Verification items for the finished model (mm, model axes). Give positions to 0.01 mm unless a question says otherwise; leave off trailing zeros. Order: outer loops, then holes, each group sorted by start corner. A loop starts at its lowest first (then second) coordinate and runs counter-clockwise, first axis right, second up.
from build123d import *

# Parameters (mm, degrees)
F0_R     = 116
F1_DEPTH = 6
F3_D     = 9.1
F5_D     = 23


with BuildPart() as f1:
    # F0 (on Top) → F1 (new body)
    with BuildSketch(Plane.XY):
        Circle(F0_R)
    extrude(amount=F1_DEPTH)

    # F3 (through all)
    with Locations(Plane.XY.offset(6)):
        with Locations((-54.4375, 94.288516), (54.4375, 94.288516), (108.875, 0), (54.4375, -94.288516), (-54.4375, -94.288516), (-108.875, 0)):
            Hole(F3_D / 2)

    # F5 (through all)
    with Locations(Plane.XY.offset(6)):
        with Locations((0, 0)):
            Hole(F5_D / 2)


solid = f1.part
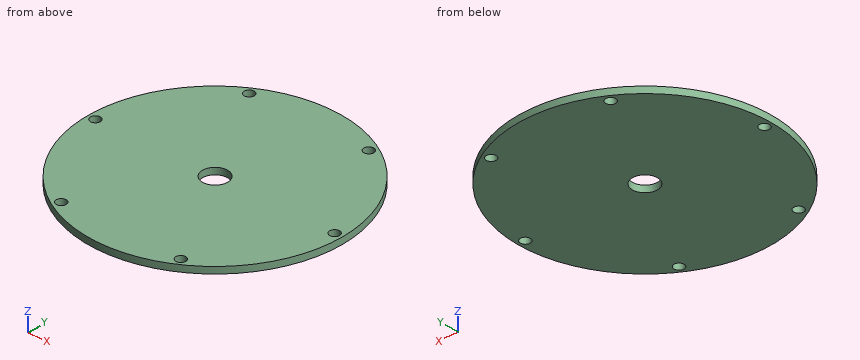
(1) Section check C-C, the plane z = 2.55. Give the number of separate pieces and of enclosed holes in the cut face, then the cut area to 3 significant figures.
Solved:
separate pieces: 1
enclosed holes: 7
area: 41,500 mm2
(2) Scan lines: line 1 (X direction, y = 91, z = 2.7); line 2 (Y direction, x = -24, z = 0.8); line 3 (Y direction, x = 106.5, z = 4.65). Record each from-to range of solid material in increasing order.
Solved:
line 1: x = -71.94 to -57.58, -51.29 to 51.29, 57.58 to 71.94
line 2: y = -113.49 to 113.49
line 3: y = -45.98 to -3.88, 3.88 to 45.98
(3) Section check A-A, the plane x = 0. Enter the section's corners in (y, z), then the cut area to 3 significant figures.
Solved:
outline: (-116, 0) - (-11.5, 0) - (-11.5, 6) - (-116, 6) - close; (11.5, 0) - (116, 0) - (116, 6) - (11.5, 6) - close
area: 1,250 mm2
(4) Section check B-B, the plane y = 0. Enter the section's corners in (x, z) (3 decimals).
Solved:
outline: (-116, 0) - (-113.425, 0) - (-113.425, 6) - (-116, 6) - close; (-104.325, 0) - (-11.5, 0) - (-11.5, 6) - (-104.325, 6) - close; (11.5, 0) - (104.325, 0) - (104.325, 6) - (11.5, 6) - close; (113.425, 0) - (116, 0) - (116, 6) - (113.425, 6) - close
(5) Go/stop test with flat-tipped pins: pin 1 (1.5 mm diameter, centred on y = 67.5, z = 5, fed in from -X); pin 2 (14 mm diameter, centred on x = 0, y = 0, fed in from +Z); pin 3 (10.5 mm diameter, centred on x = 54.44, y = 94.29, fed in from -Z); pin 4 (2 mm diameter, centred on x = 70, z = 2.5, fed in from +Y). Record where each tip stops, or that it passes through.
Solved:
pin 1: stops at x = -94.87
pin 2: passes through
pin 3: stops at z = 0
pin 4: stops at y = 93.25
(6) Section check D-D, the plane y = -44.5. Enter the section's corners in (x, z).
Solved:
outline: (-107.12, 0) - (107.12, 0) - (107.12, 6) - (-107.12, 6) - close
